For this review, take the finished solid that the model builds, in its own axes (mm). A direction names the side the tool comes from. Coordinates: 2 decimals unless noted, no trailing zeros. Order: outer loops, then holes, each group sorted by start corner. A loop starts at its lowest first (then second) coordinate and runs counter-clockwise, first axis right, second up. Notation, with made-up numbers: (-2.75, -28.75) -> (14.25, -28.75) arc R12 ccw to (14.25, -20.75) -> close; hole circle Ø1 at (39.5, 9). An arc over 180 degrees is marked (long way). Write item = value, one per line. Start each with the question number.
1) Consider section D-D on y = 33.5. Give the boundary of the cut face in (x, z), and give its area (3 significant figures).
2) Consider section A-A on y = 42. Give the boundary of the cut face in (x, z) (3 decimals).
3) Wall thickness on probe 1 along X at (y, z) = (-13.5, 6.35); probe 2 along X at (y, z) = (-22, 6.65); probe 3 along X at (y, z) = (-22, 2.9): over which ranges is each line inside the solid? List them lowest first. Write a range as [from, to].
4) Machinability: for faces 1 (the face through (-43.6, 38.8, 2)), 2 (the face through (75.486, 44.297, 4.056)), which of the approach directions +Z, -Z, +X, -X, +Y, -Y give a long, thin tool a straight path to every point of the face, cutting with its end or side? Answer none if there is none.
5) Insertion check: pin 1 Ø7 at (x, y) = (-46, 42) entering from -Z; pin 2 Ø1.6 at (x, y) = (-43, 13) entering from -Z; pin 3 Ø1.7 at (x, y) = (-41.5, -13.5) entering from -Z. Each pin has a flat end and moves straight along its axis. Give the tip position at first contact, or say it passes through.
6) Draft analysis for pull direction X (two halves, no side actions). For faces 3 (the face through (13, 11, 8)), 4 (the face through (81.5, 0, 4)), 5 (the face through (51, 35, 2)), 6 (the face through (-53.5, 9, 4)), state which applies: +X half, -X half, draft (parallel to the pull), parting line (faces both ways), or undercut.
7) Consider section C-C on y = -22. State how many separate pieces and enclosed holes the cut face has, and give its area (3 significant figures).
8) Consider section B-B on x = -46. Give the boundary of the cut face in (y, z) (3 decimals), and give its area (3 significant figures).
from build123d import *

# Parameters (mm, degrees)
SKETCH1_W                       = 135
SKETCH1_H                       = 80
BOSS_EXTRUDE1_DEPTH             = 8
CBORE_FOR_M2_5_SHCS1_AT_2_COUNT = 2
CBORE_FOR_M2_5_SHCS1_AT_2_PITCH = 27
CBORE_FOR_M2_5_SHCS1_AT_3_COUNT = 2
CBORE_FOR_M2_5_SHCS1_AT_3_PITCH = 58.591808301
CBORE_FOR_M2_5_SHCS1_AT_4_COUNT = 2
CBORE_FOR_M2_5_SHCS1_AT_4_PITCH = 52
CBORE_FOR_M4_SHCS3_AT_2_COUNT   = 2
CBORE_FOR_M4_SHCS3_AT_2_PITCH   = 60
CBORE_FOR_M4_SHCS3_AT_3_COUNT   = 2
CBORE_FOR_M4_SHCS3_AT_3_PITCH   = 120
CBORE_FOR_M4_SHCS3_AT_4_COUNT   = 2
CBORE_FOR_M4_SHCS3_AT_4_PITCH   = 64
CBORE_FOR_M4_SHCS3_AT_5_COUNT   = 2
CBORE_FOR_M4_SHCS3_AT_5_PITCH   = 87.726848798
FILLET1_R                       = 20


with BuildPart() as part:
    # Sketch1 → Boss-Extrude1 (new body)
    with BuildSketch(Plane.XY):
        with Locations((14, 10)):
            Rectangle(SKETCH1_W, SKETCH1_H)
    extrude(amount=BOSS_EXTRUDE1_DEPTH)

    # Sketch4 → CBORE for M2.5 SHCS1 (revolve, cut)
    with BuildSketch(Plane(origin=(10.5, 13.5, 0), x_dir=(0, 1, 0), z_dir=(1, 0, 0))):
        Polygon((0, 0), (0, 8), (1.45, 8), (1.45, 2.5), (2.75, 2.5), (2.75, 0.025), (2.775, 0), align=None)
    cbore_for_m2_5_shcs1 = revolve(axis=Axis((10.5, 13.5, -6.35), (0, 0, 1)), mode=Mode.SUBTRACT)

    # CBORE for M2.5 SHCS1 at 2: CBORE for M2.5 SHCS1 ×2
    with Locations(*[(0, -i * CBORE_FOR_M2_5_SHCS1_AT_2_PITCH, 0) for i in range(1, CBORE_FOR_M2_5_SHCS1_AT_2_COUNT)]):
        add(cbore_for_m2_5_shcs1, mode=Mode.SUBTRACT)

    # CBORE for M2.5 SHCS1 at 3: CBORE for M2.5 SHCS1 ×2
    with Locations(*[Vector(-0.8874960768017397, -0.4608152706470572, 0) * (i * CBORE_FOR_M2_5_SHCS1_AT_3_PITCH) for i in range(1, CBORE_FOR_M2_5_SHCS1_AT_3_COUNT)]):
        add(cbore_for_m2_5_shcs1, mode=Mode.SUBTRACT)

    # CBORE for M2.5 SHCS1 at 4: CBORE for M2.5 SHCS1 ×2
    with Locations(*[(-i * CBORE_FOR_M2_5_SHCS1_AT_4_PITCH, 0, 0) for i in range(1, CBORE_FOR_M2_5_SHCS1_AT_4_COUNT)]):
        add(cbore_for_m2_5_shcs1, mode=Mode.SUBTRACT)

    # Sketch5 → Cut-Revolve1 (revolve, cut)
    with BuildSketch(Plane(origin=(60, 0, 0), x_dir=(0, 0, -1), z_dir=(1, 0, 0)), mode=Mode.PRIVATE) as cut_revolve1_sk:
        Polygon((-8, 39.5), (-2, 39.5), (-2, 38.5), (0, 38.5), (0, 26), (-8, 26), align=None)
    revolve(cut_revolve1_sk.sketch.rotate(Axis((60, 26, 0), (0, 0, 1)), 90), axis=Axis((60, 26, 0), (0, 0, 1)), mode=Mode.SUBTRACT)

    # Sketch17 → CBORE for M4 SHCS3 (revolve, cut)
    with BuildSketch(Plane(origin=(-46, -22, 0), x_dir=(0, 1, 0), z_dir=(1, 0, 0))):
        Polygon((0, 0), (0, 8), (2.25, 8), (2.25, 4), (4, 4), (4, 0.025), (4.025, 0), align=None)
    cbore_for_m4_shcs3 = revolve(axis=Axis((-46, -22, -6.35), (0, 0, 1)), mode=Mode.SUBTRACT)

    # CBORE for M4 SHCS3 at 2: CBORE for M4 SHCS3 ×2
    with Locations(*[(i * CBORE_FOR_M4_SHCS3_AT_2_PITCH, 0, 0) for i in range(1, CBORE_FOR_M4_SHCS3_AT_2_COUNT)]):
        add(cbore_for_m4_shcs3, mode=Mode.SUBTRACT)

    # CBORE for M4 SHCS3 at 3: CBORE for M4 SHCS3 ×2
    with Locations(*[(i * CBORE_FOR_M4_SHCS3_AT_3_PITCH, 0, 0) for i in range(1, CBORE_FOR_M4_SHCS3_AT_3_COUNT)]):
        add(cbore_for_m4_shcs3, mode=Mode.SUBTRACT)

    # CBORE for M4 SHCS3 at 4: CBORE for M4 SHCS3 ×2
    with Locations(*[(0, i * CBORE_FOR_M4_SHCS3_AT_4_PITCH, 0) for i in range(1, CBORE_FOR_M4_SHCS3_AT_4_COUNT)]):
        add(cbore_for_m4_shcs3, mode=Mode.SUBTRACT)

    # CBORE for M4 SHCS3 at 5: CBORE for M4 SHCS3 ×2
    with Locations(*[Vector(0.6839411288813297, 0.7295372041400852, 0) * (i * CBORE_FOR_M4_SHCS3_AT_5_PITCH) for i in range(1, CBORE_FOR_M4_SHCS3_AT_5_COUNT)]):
        add(cbore_for_m4_shcs3, mode=Mode.SUBTRACT)

    # Fillet1
    fillet1_edges = [part.edges().sort_by_distance(p)[0] for p in [
        (81.5, 50, 4),
    ]]
    fillet(fillet1_edges, radius=FILLET1_R)


solid = part.part
Answer sheet:
q1.outline = (-53.5, 0) -> (50, 0) -> (50, 2) -> (48.78, 2) -> (48.78, 8) -> (-53.5, 8) -> close; (70, 0) -> (81.19, 0) -> (81.19, 8) -> (71.22, 8) -> (71.22, 2) -> (70, 2) -> close
q1.area = 903 mm2
q2.outline = (-53.5, 0) -> (-50.025, 0) -> (-50, 0.025) -> (-50, 4) -> (-48.25, 4) -> (-48.25, 8) -> (-53.5, 8) -> close; (-43.75, 4) -> (-42, 4) -> (-42, 0.025) -> (-41.975, 0) -> (9.975, 0) -> (10, 0.025) -> (10, 4) -> (11.75, 4) -> (11.75, 8) -> (-43.75, 8) -> close; (16.25, 4) -> (18, 4) -> (18, 0.025) -> (18.025, 0) -> (77.5, 0) -> (77.5, 8) -> (16.25, 8) -> close
q3.probe_1 = [-53.5, -42.95], [-40.05, 9.05], [11.95, 81.5]
q3.probe_2 = [-53.5, -48.25], [-43.75, 11.75], [16.25, 71.75], [76.25, 81.5]
q3.probe_3 = [-53.5, -50], [-42, 10], [18, 70], [78, 81.5]
q4.face_1 = -Z
q4.face_2 = +Z, -Z, +X, +Y
q5.pin_1 = 4
q5.pin_2 = 2.5
q5.pin_3 = through
q6.face_3 = draft
q6.face_4 = +X half
q6.face_5 = undercut
q6.face_6 = -X half
q7.separate_pieces = 4
q7.enclosed_holes = 0
q7.area = 930 mm2
q8.outline = (-30, 0) -> (-26.025, 0) -> (-26, 0.025) -> (-26, 4) -> (-24.25, 4) -> (-24.25, 8) -> (-30, 8) -> close; (-19.75, 4) -> (-18, 4) -> (-18, 0.025) -> (-17.975, 0) -> (37.975, 0) -> (38, 0.025) -> (38, 4) -> (39.75, 4) -> (39.75, 8) -> (-19.75, 8) -> close; (44.25, 4) -> (46, 4) -> (46, 0.025) -> (46.025, 0) -> (50, 0) -> (50, 8) -> (44.25, 8) -> close
q8.area = 540 mm2
